```python
from build123d import *

# Parameters (mm, degrees)
SKETCH_W        = 1346.2
SKETCH_H        = 622.3
PAD_DEPTH       = 18.669
POCKET_DEPTH    = 18.67
POCKET001_DEPTH = 18.67
SKETCH003_W     = 63.5
SKETCH003_H     = 76.2
PAD001_DEPTH    = 18.669
FILLET_R        = 12.7
FILLET001_R     = 127
SKETCH004_W     = 30.48
SKETCH004_H     = 30.48
POCKET002_DEPTH = 18.67
SKETCH005_R     = 4.490128
POCKET003_DEPTH = 18.67
FILLET002_R     = 127
FILLET003_R     = 127
FILLET004_R     = 76.2
SKETCH006_W     = 736.6
SKETCH006_H     = 762
POCKET004_DEPTH = 18.67
SKETCH007_R     = 6.35
POCKET005_DEPTH = 2.54


with BuildPart() as part:
    # Sketch → Pad (new body)
    with BuildSketch(Plane.XY):
        Rectangle(SKETCH_W, SKETCH_H)
    extrude(amount=PAD_DEPTH)

    # Sketch001 (on Face6 of Pad) → Pocket (cut, through all)
    with BuildSketch(Plane.XY.offset(18.669)):
        Polygon((-355.6, -120.65), (355.6, -120.65), (469.9, -311.15), (-469.9, -311.15), align=None)
    extrude(amount=-POCKET_DEPTH, mode=Mode.SUBTRACT)

    # Sketch002 (on Face5 of Pocket) → Pocket001 (cut, through all)
    with BuildSketch(Plane.XY.offset(18.669)):
        Polygon((-342.9, 311.15), (342.9, 311.15), (203.2, 158.75), (-203.2, 158.75), align=None)
    extrude(amount=-POCKET001_DEPTH, mode=Mode.SUBTRACT)

    # Sketch003 (on Face4 of Pocket001) → Pad001 (join)
    with BuildSketch(Plane.XY.offset(18.669)):
        with Locations((704.85, 77.47)):
            Rectangle(SKETCH003_W, SKETCH003_H)
        with Locations((704.85, -74.93)):
            Rectangle(SKETCH003_W, SKETCH003_H)
        with Locations((704.85, -227.33)):
            Rectangle(SKETCH003_W, SKETCH003_H)
        with Locations((-704.85, -227.33)):
            Rectangle(SKETCH003_W, SKETCH003_H)
        with Locations((-704.85, 77.47)):
            Rectangle(SKETCH003_W, SKETCH003_H)
        with Locations((-704.85, -74.93)):
            Rectangle(SKETCH003_W, SKETCH003_H)
    extrude(amount=-PAD001_DEPTH)

    # Fillet
    fillet_edges = [part.edges().sort_by_distance(p)[0] for p in [
        (673.1, -311.15, 9.3345),
        (-673.1, -311.15, 9.3345),
        (-469.9, -311.15, 9.3345),
        (469.9, -311.15, 9.3345),
    ]]
    fillet(fillet_edges, radius=FILLET_R)

    # Fillet001
    fillet001_edges = [part.edges().sort_by_distance(p)[0] for p in [
        (-673.1, 311.15, 9.3345),
        (673.1, 311.15, 9.3345),
    ]]
    fillet(fillet001_edges, radius=FILLET001_R)

    # Sketch004 (on Face52 of Fillet001) → Pocket002 (cut, through all)
    with BuildSketch(Plane.XY.offset(18.669)):
        with Locations((-688.34, 54.61)):
            Rectangle(SKETCH004_W, SKETCH004_H)
        with Locations((-688.34, -97.79)):
            Rectangle(SKETCH004_W, SKETCH004_H)
        with Locations((-688.34, -250.19)):
            Rectangle(SKETCH004_W, SKETCH004_H)
        with Locations((688.34, -250.19)):
            Rectangle(SKETCH004_W, SKETCH004_H)
        with Locations((688.34, -97.79)):
            Rectangle(SKETCH004_W, SKETCH004_H)
        with Locations((688.34, 54.61)):
            Rectangle(SKETCH004_W, SKETCH004_H)
    extrude(amount=-POCKET002_DEPTH, mode=Mode.SUBTRACT)

    # Sketch005 (on Face69 of Pocket002) → Pocket003 (cut, through all)
    with BuildSketch(Plane.XY.offset(18.669)):
        with Locations((703.58, -234.95)):
            Circle(SKETCH005_R)
        with Locations((673.1, -234.95)):
            Circle(SKETCH005_R)
        with Locations((703.58, -82.55)):
            Circle(SKETCH005_R)
        with Locations((673.1, -82.55)):
            Circle(SKETCH005_R)
        with Locations((703.58, 69.85)):
            Circle(SKETCH005_R)
        with Locations((673.1, 69.85)):
            Circle(SKETCH005_R)
        with Locations((-673.1, 69.85)):
            Circle(SKETCH005_R)
        with Locations((-703.58, 69.85)):
            Circle(SKETCH005_R)
        with Locations((-673.1, -82.55)):
            Circle(SKETCH005_R)
        with Locations((-703.58, -82.55)):
            Circle(SKETCH005_R)
        with Locations((-703.58, -234.95)):
            Circle(SKETCH005_R)
        with Locations((-673.1, -234.95)):
            Circle(SKETCH005_R)
    extrude(amount=-POCKET003_DEPTH, mode=Mode.SUBTRACT)

    # Fillet002
    fillet002_edges = [part.edges().sort_by_distance(p)[0] for p in [
        (-355.6, -120.65, 9.3345),
        (355.6, -120.65, 9.3345),
    ]]
    fillet(fillet002_edges, radius=FILLET002_R)

    # Fillet003
    fillet003_edges = [part.edges().sort_by_distance(p)[0] for p in [
        (-342.9, 311.15, 9.3345),
        (342.9, 311.15, 9.3345),
    ]]
    fillet(fillet003_edges, radius=FILLET003_R)

    # Fillet004
    fillet004_edges = [part.edges().sort_by_distance(p)[0] for p in [
        (-203.2, 158.75, 9.3345),
        (203.2, 158.75, 9.3345),
    ]]
    fillet(fillet004_edges, radius=FILLET004_R)

    # Sketch006 (on Face53 of Fillet004) → Pocket004 (cut, through all)
    with BuildSketch(Plane.XY.offset(18.669)):
        with Locations((-368.3, 0)):
            Rectangle(SKETCH006_W, SKETCH006_H)
    extrude(amount=-POCKET004_DEPTH, mode=Mode.SUBTRACT)

    # Sketch007 (on Face28 of Pocket004) → Pocket005 (cut)
    with BuildSketch(Plane.XY.offset(18.669)):
        with Locations((76.2, -82.55)):
            Circle(SKETCH007_R)
        with Locations((228.6, -82.55)):
            Circle(SKETCH007_R)
        with Locations((381, -82.55)):
            Circle(SKETCH007_R)
        with Locations((533.4, -82.55)):
            Circle(SKETCH007_R)
    extrude(amount=-POCKET005_DEPTH, mode=Mode.SUBTRACT)


with BuildPart() as part_1:
    # Clone placement: moved
    add(part.part.moved(Location((0, 0, -18.669))))


solid = part_1.part
```
The model under review builds one solid part; all positions refer to its coordinate system, in mm. A direction names the side the tool comes from. Round coordinates to 2 decimals unless told otherwise and drop trailing zeros. Write each loop counter-clockwise with the first axis right and the second up, starting at its lowest first coordinate (ties: lowest second). Pieces come first, ordered by that corner, then holes.
(1) Insertion check: pin 1 (4 mm diameter, centred on x = 78.5, y = -83.5, fed in from +Z); pin 2 (6 mm diameter, centred on x = 470.5, z = -7, fed in from -Y); pin 3 (9.5 mm diameter, centred on x = 699, z = -11, fed in from +Y). Each pin has a flat end and moves straight along its axis. Give the tip position at first contact, or say it passes through.
(2) We need section B-B on x = 58.5. Give the boundary of the cut face in (y, z).
(3) Mouldability with a two-part tool opening along Y and no side actions: class faces 4 (the flat face through (266.055, 227.319, -9.204)), 5 (the flat face through (673.1, 14, -9)), 6 (the flat face through (736.6, -228, -9)), 7 (the flat face through (428.883, -242.788, -9.204)) as +Y half, -Y half, draft (parallel to the pull), parting line (faces both ways), or undercut.
(4) Machinability: for faces 1 (the flat face through (703.58, -253, -9)), 2 (the flat face through (720, -265.43, -9)), 3 (the flat face through (703.58, -100, -9)), which of the approach directions +Z, -Z, +X, -X, +Y, -Y give a long, thin tool a straight path to every point of the face, cutting with its end or side? Answer none if there is none.
(5) We need section A-A on y = -218.5. Give the boundary of the cut face in (x, z), and give its area (3 significant figures).
(6) Wall thickness on L1, parallel to X at y = 58, z = -9.5; L2, parallel to Y at x = 76.2, z = -0.7; L3, parallel to Y at x = 381, z = -1.05: over which ranges is each line inside the solid? List them lowest first.
Findings below:
1. pin 1: stops at z = -2.54
1. pin 2: stops at y = -310.63
1. pin 3: stops at y = 115.57
2. outline: (-120.65, -18.67) - (158.75, -18.67) - (158.75, 0) - (-120.65, 0) - close
3. face 4: +Y half
3. face 5: undercut
3. face 6: draft
3. face 7: -Y half
4. face 1: +Z, -Z, -Y
4. face 2: +Z, -Z, +X, -Y
4. face 3: +Z, -Z
5. outline: (414.31, -18.67) - (736.6, -18.67) - (736.6, 0) - (414.31, 0) - close
5. area: 6,020 mm2
6. L1: x = 0 to 673.1, 703.58 to 736.6
6. L2: y = -120.65 to -88.9, -76.2 to 158.75
6. L3: y = -166.04 to -88.9, -76.2 to 309.9
